from build123d import *

# Parameters (mm, degrees)
BASE_FLANGE1_DEPTH = 100
SKETCH6_R          = 17.5
CUT_EXTRUDE1_DEPTH = 10
FILLET1_R          = 5
FILLET2_R          = 5
SKETCH7_R          = 3
CUT_EXTRUDE2_DEPTH = 10
CUT_EXTRUDE3_DEPTH = 10


# Sheet-metal steps are written as plain solids
with BuildPart() as part:
    # Sketch1 → Base-Flange1 (new body)
    with BuildSketch(Plane.XY):
        with BuildLine():
            Line((0, 84.5), (0, 4))
            ThreePointArc((0, 4), (-1.171572875, 1.171572875), (-4, 0))
            Line((-4, 0), (-30, 0))
            Line((-30, 0), (-30, 2))
            Line((-30, 2), (-4, 2))
            ThreePointArc((-4, 2), (-2.585786438, 2.585786438), (-2, 4))
            Line((-2, 4), (-2, 84.5))
            Line((-2, 84.5), (0, 84.5))
        make_face()
    extrude(amount=BASE_FLANGE1_DEPTH)

    # Sketch6 → Cut-Extrude1 (cut)
    with BuildSketch(Plane.ZY.offset(2)):
        with Locations((50, 84.5)):
            Circle(SKETCH6_R)
    extrude(amount=-CUT_EXTRUDE1_DEPTH, mode=Mode.SUBTRACT)

    # Fillet1
    fillet1_edges = [part.edges().sort_by_distance(p)[0] for p in [
        (-1, 84.5, 100),
        (-1, 84.5, 32.5),
        (-1, 84.5, 67.5),
        (-1, 84.5, 0),
    ]]
    fillet(fillet1_edges, radius=FILLET1_R)

    # Fillet2
    fillet2_edges = [part.edges().sort_by_distance(p)[0] for p in [
        (-30, 1, 100),
        (-30, 1, 0),
    ]]
    fillet(fillet2_edges, radius=FILLET2_R)

    # Sketch7 → Cut-Extrude2 (cut)
    with BuildSketch(Plane(origin=(0, 2, 0), x_dir=(1, 0, 0), z_dir=(0, 1, 0))):
        with Locations(Location((-15, -25, 0), (0, 0, 270))):
            Circle(SKETCH7_R)
        with Locations(Location((-15, -75, 0), (0, 0, 270))):
            Circle(SKETCH7_R)
    extrude(amount=-CUT_EXTRUDE2_DEPTH, mode=Mode.SUBTRACT)

    # Sketch8 → Cut-Extrude3 (cut)
    with BuildSketch(Plane.ZY.offset(2)):
        with BuildLine():
            Line((21.5, 72), (21.5, 59))
            ThreePointArc((21.5, 59), (25, 55.5), (28.5, 59))
            Line((28.5, 59), (28.5, 72))
            ThreePointArc((28.5, 72), (25, 75.5), (21.5, 72))
        make_face()
        with BuildLine():
            Line((78.5, 72), (78.5, 59))
            ThreePointArc((78.5, 59), (75, 55.5), (71.5, 59))
            Line((71.5, 59), (71.5, 72))
            ThreePointArc((71.5, 72), (75, 75.5), (78.5, 72))
        make_face()
    extrude(amount=-CUT_EXTRUDE3_DEPTH, mode=Mode.SUBTRACT)


solid = part.part
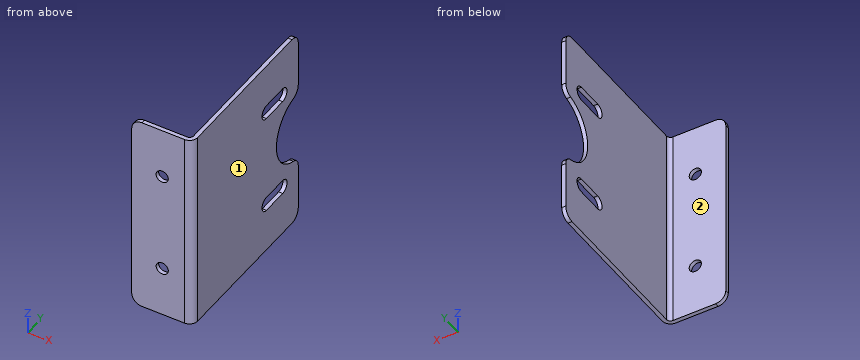
Build history of the part. All positions in model axes, mm. Face numbers are marked on the shaded views. A direction names the side the tool comes from. Round coordinates to 2 decimals unless told otherwise and drop trailing zeros. Write each loop counter-clockwise with the first axis right and the second up, starting at its lowest first coordinate (ties: lowest second). Pieces come first, ordered by that corner, then holes. Notation, with made-up numbers: M 7.5,-9.75 L 60.5,-9.75 A14 ccw 60.5,-5.75 Z; hole C 55,-24 d1. An arc over 180 degrees is marked long. Use CSV: the item, a comma, the result in double quotes.
1. Saw through at B-B (z = 75). Give the cut face in (x, y).
Reply:
outline,"M -30,0 L -18,0 L -18,2 L -30,2 Z; M -12,0 L -4,0 A4 ccw 0,4 L 0,55.5 L -2,55.5 L -2,4 A2 cw -4,2 L -12,2 Z; M -2,75.5 L 0,75.5 L 0,84.5 L -2,84.5 Z"
2. Tool access for the marked faces 1 and 2: list every direction of +Z, -Z, +X, -X, +Y, -Y with a clear straight run to the whole face (end or side of a thin tool).
Reply:
face 1,"+Z, -Z, +X, +Y, -Y"
face 2,"+Z, -Z, -X, +Y"
3. Saw through at A-A (x = -15). Give the cut face in (y, z), plus the area to 3 significant figures.
Reply:
outline,"M 0,0 L 2,0 L 2,22 L 0,22 Z; M 0,28 L 2,28 L 2,72 L 0,72 Z; M 0,78 L 2,78 L 2,100 L 0,100 Z"
area,"176 mm²"
4. Saw through at C-C (y = 13). Give the cut face in (x, z), plus the area to 3 significant figures.
Reply:
outline,"M -2,0 L 0,0 L 0,100 L -2,100 Z"
area,"200 mm²"
5. Wall check: probe 1 along Y at (x, z) = (-19.25, 14); probe 2 along X at (y, z) = (1, 75); probe 3 along X at (y, z) = (8, 39). Give the ranges that are in metal, low to high. Write a range as from..to.
Reply:
probe 1,"y = 0..2"
probe 2,"x = -30..-18, -12..-1.35"
probe 3,"x = -2..0"
6. Flat gauge pins, fed straight in: pin 1 (3 mm diameter, centred on y = 63, z = 44.5, fed in from -X); pin 2 (10 mm diameter, centred on x = -16, z = 70, fed in from +Y). Where does each tip first touch, or does it go through?
Reply:
pin 1,"stops at x = -2"
pin 2,"stops at y = 2"
